Design review of the part built by this model. Coordinates are the model's own, in mm. A direction names the side the tool comes from. Coordinates: 2 decimals unless noted, no trailing zeros. Loops run counter-clockwise (first coordinate to the right, second up) from the corner with the lowest first, then second, coordinate; pieces in that order, holes last. Notation, with made-up numbers: M 87.25,-33.5 L 130.25,-33.5 A10 ccw 130.25,-26.5 Z; hole C 28,88.25 d5. An arc over 180 degrees is marked long. Answer as a JSON object with one key per item and string values. Group by question number.
1. Consider section C-C (y = -113.5). State the section outline as (x, z) points.
2. Consider section B-B (x = 26). State the section outline as (y, z) points, then the cut area to 3 significant figures.
3. To check wall thickness, follow probe 1 along Y at (x, z) = (55, 33); probe 2 along Z at (x, y) = (219, -110); probe 3 along Z at (x, y) = (252, -110). State the ranges of each line that lie inside material, in increasing order.
4. Consider section A-A (z = 33). State the section outline as (x, y) points.
5. Consider section D-D (y = -64). State the section outline as (x, z) points, then the cut area to 4 significant figures.
6. Draft analysis for pull direction X (two halves, no side actions). For faces 5 (the flat face through (137, -26, 78.5)), 6 (the flat face through (124, -110, 45)), 7 (the flat face through (270, -108, 49)), state which applies: +X half, -X half, draft (parallel to the pull), parting line (faces both ways), or undercut.
7. Insertion check: pin 1 (10 mm diameter, centred on x = 124, y = -113, fed in from -Z); pin 2 (2 mm diameter, centred on x = 143, y = -108.5, fed in from +Z); pin 3 (12 mm diameter, centred on x = 73, y = -29, fed in from -Z); pin 4 (9.5 mm diameter, centred on y = -110, z = 33, fed in from +X). Each pin has a flat end and moves straight along its axis. Give the tip position at first contact, or say it passes through.
8. Machinability: for faces 1 (the cylindrical face through (253, -118, 27)), 2 (the flat face through (133, -109, 52.5)), 3 (the flat face through (126, -120, 32)), 4 (the flat face through (10, -101, 33)), which of the approach directions +Z, -Z, +X, -X, +Y, -Y give a long, thin tool a straight path to every point of the face, cutting with its end or side? Answer none if there is none.
from build123d import *

# Parameters (mm, degrees)
F1_DEPTH  = 220
F2_R      = 8
F3_DEPTH  = 270.001
F2_R_2    = 10
F4_DEPTH  = 35
F6_DEPTH  = 25
F8_DEPTH  = 10
F9_W      = 115
F9_H      = 26
F10_DEPTH = 270.001


with BuildPart() as f1:
    # F0 (on Front) → F1 (new body)
    with BuildSketch(Plane.XZ):
        Polygon((0, 78.5), (0, 0), (20, 0), (20, 20), (270, 20), (270, 78.5), align=None)
    extrude(amount=F1_DEPTH)

    # F2 (on face) → F3 (cut, through all)
    with BuildSketch(Plane.YZ.offset(270)):
        with Locations((-110, 33)):
            Circle(F2_R)
    extrude(amount=-F3_DEPTH, mode=Mode.SUBTRACT)

    # F2 (on face) → F4 (cut)
    with BuildSketch(Plane.YZ.offset(270)):
        with Locations((-110, 33)):
            Circle(F2_R_2)
        with Locations((-110, 33)):
            Circle(F2_R, mode=Mode.SUBTRACT)
    extrude(amount=-F4_DEPTH, mode=Mode.SUBTRACT)

    # F5 (on face) → F6 (cut)
    with BuildSketch(Plane(origin=(0, 0, 20), x_dir=(1, 0, 0), z_dir=(0, 0, -1))):
        with BuildLine():
            Line((165, 120), (85, 120))
            ThreePointArc((85, 120), (75, 110), (85, 100))
            Line((85, 100), (165, 100))
            ThreePointArc((165, 100), (175, 110), (165, 120))
        make_face()
    extrude(amount=-F6_DEPTH, mode=Mode.SUBTRACT)

    # F7 (on face) → F8 (cut)
    with BuildSketch(Plane(origin=(0, 0, 0), x_dir=(0, -1, 0), z_dir=(-1, 0, 0))):
        with BuildLine():
            Line((117, 42), (101, 42))
            ThreePointArc((101, 42), (92, 33), (101, 24))
            Line((101, 24), (117, 24))
            ThreePointArc((117, 24), (126, 33), (117, 42))
        make_face()
    extrude(amount=-F8_DEPTH, mode=Mode.SUBTRACT)

    # F9 (on face) → F10 (cut, through all)
    with BuildSketch(Plane(origin=(0, 0, 0), x_dir=(0, -1, 0), z_dir=(-1, 0, 0))):
        with Locations((110, 65.5)):
            Rectangle(F9_W, F9_H)
    extrude(amount=-F10_DEPTH, mode=Mode.SUBTRACT)


solid = f1.part
Findings below:
{
 "1": {"outline": "M 0,0 L 20,0 L 20,20 L 75.63,20 L 75.63,25.81 L 10,25.81 L 10,24 L 0,24 Z; M 0,42 L 10,42 L 10,40.19 L 75.63,40.19 L 75.63,45 L 174.37,45 L 174.37,40.19 L 235,40.19 L 235,42.37 L 270,42.37 L 270,52.5 L 0,52.5 Z; M 174.37,20 L 270,20 L 270,23.63 L 235,23.63 L 235,25.81 L 174.37,25.81 Z"},
 "2": {"outline": "M -220,20 L 0,20 L 0,78.5 L -52.5,78.5 L -52.5,52.5 L -167.5,52.5 L -167.5,78.5 L -220,78.5 Z; hole C -110,33 d16", "area": "9,680 mm^2"},
 "3": {"probe 1": "y = -220 to -118, -102 to 0", "probe 2": "z = 20 to 25, 41 to 52.5", "probe 3": "z = 20 to 23, 43 to 52.5"},
 "4": {"outline": "M 0,-220 L 270,-220 L 270,-120 L 235,-120 L 235,-118 L 171,-118 A10 cw 165,-120 L 85,-120 A10 cw 79,-118 L 10,-118 L 10,-126 L 0,-126 Z; M 0,-92 L 10,-92 L 10,-102 L 79,-102 A10 cw 85,-100 L 165,-100 A10 cw 171,-102 L 235,-102 L 235,-100 L 270,-100 L 270,0 L 0,0 Z"},
 "5": {"outline": "M 0,0 L 20,0 L 20,20 L 270,20 L 270,52.5 L 0,52.5 Z", "area": "9,175 mm^2"},
 "6": {"face 5": "draft", "face 6": "undercut", "face 7": "+X half"},
 "7": {"pin 1": "stops at z = 45", "pin 2": "stops at z = 52.5", "pin 3": "stops at z = 20", "pin 4": "passes through"},
 "8": {"face 1": "+X", "face 2": "+Z, +X, -X", "face 3": "-Z", "face 4": "-X"}
}
